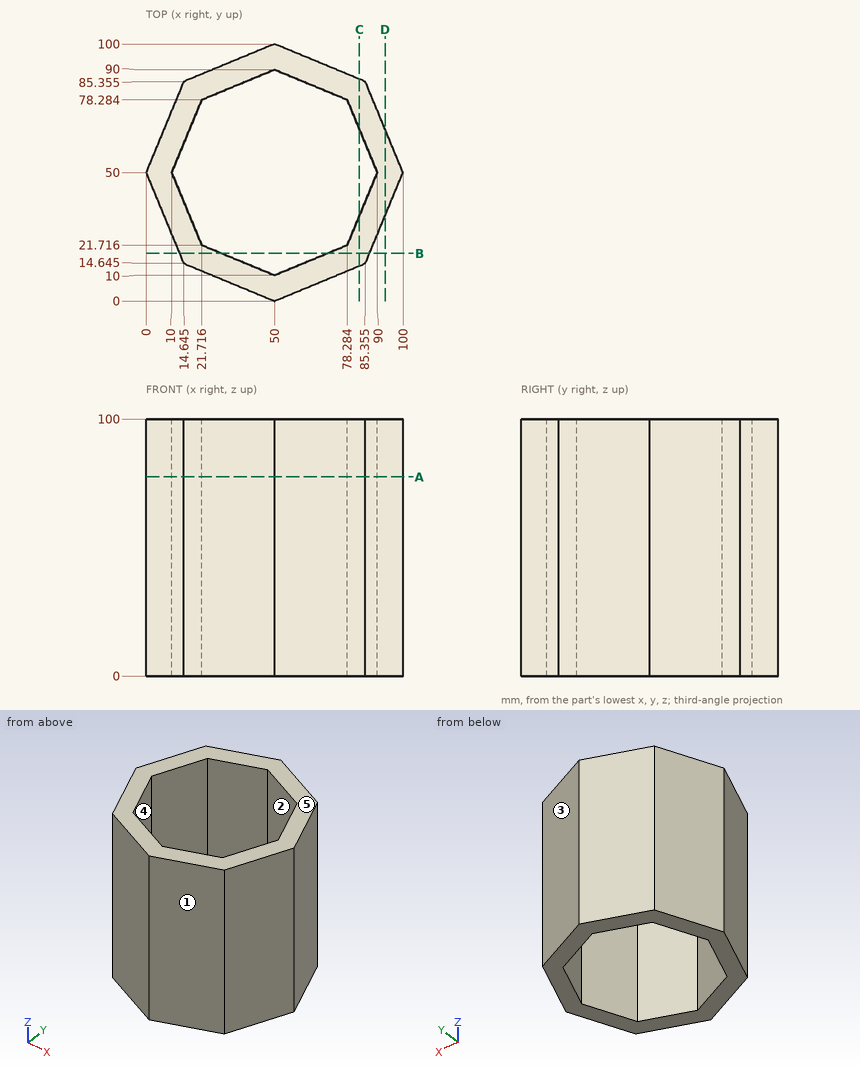
The drawing under review shows one solid part. Ordinate dimensions are in mm from its lowest x, y, z. A direction names the side the tool comes from. Round coordinates to 2 decimals unless told otherwise and drop trailing zeros. Loops run counter-clockwise (first coordinate to the right, second up) from the corner with the lowest first, then second, coordinate; pieces in that order, holes last. Notation, with made-up numbers: (15, 82.25) -> (20, 82.25) arc R23 ccw to (20, 101.25) -> close; hole circle Ø8 at (-11.75, 12). An arc over 180 degrees is marked (long way). Answer in a Markdown table with one row per item.
1) Consider section D-D, the plane x = 93. Write out the cut boundary in (y, z).
Taken from the geometry:
| item | result |
|---|---|
| outline | (33.1, 0) -> (66.9, 0) -> (66.9, 100) -> (33.1, 100) -> close |
2) Tool access review of the marked faces 1 and 2: name each direction out of +Z, -Z, +X, -X, +Y, -Y from which nothing blocks a thin tool from reaching the whole face with its end or side.
Taken from the geometry:
| item | result |
|---|---|
| face 1 | +Z, -Z, +X, -Y |
| face 2 | +Z, -Z |
3) Consider section C-C, the plane x = 83. Write out the cut boundary in (y, z).
Taken from the geometry:
| item | result |
|---|---|
| outline | (13.67, 0) -> (33.1, 0) -> (33.1, 100) -> (13.67, 100) -> close; (66.9, 0) -> (86.33, 0) -> (86.33, 100) -> (66.9, 100) -> close |
4) Consider section B-B, the plane y = 18.5. Write out the cut boundary in (x, z), plus the area to 3 significant figures.
Taken from the geometry:
| item | result |
|---|---|
| outline | (13.05, 0) -> (29.48, 0) -> (29.48, 100) -> (13.05, 100) -> close; (70.52, 0) -> (86.95, 0) -> (86.95, 100) -> (70.52, 100) -> close |
| area | 3,290 mm² |
5) Consider section A-A, the plane z = 77.5. Write out the cut boundary in (x, y) (1 decimal).
Taken from the geometry:
| item | result |
|---|---|
| outline | (0, 50) -> (14.6, 14.6) -> (50, 0) -> (85.4, 14.6) -> (100, 50) -> (85.4, 85.4) -> (50, 100) -> (14.6, 85.4) -> close; hole (10, 50) -> (21.7, 21.7) -> (50, 10) -> (78.3, 21.7) -> (90, 50) -> (78.3, 78.3) -> (50, 90) -> (21.7, 78.3) -> close |
6) Wall thickness on line 1 along Y through (x, z) = (37, 5.5) (1 decimal); line 2 along X through (y, z) = (48, 59); line 3 along Y through (x, z) = (13, 43.5) (1 decimal): over which ranges is each line inside the solid? List them lowest first.
Taken from the geometry:
| item | result |
|---|---|
| line 1 | y = 5.4 to 15.4, 84.6 to 94.6 |
| line 2 | x = 0.83 to 10.83, 89.17 to 99.17 |
| line 3 | y = 18.6 to 42.8, 57.2 to 81.4 |
7) Draft analysis for pull direction Y (two halves, no side actions). For the marked faces 3, 4 and 5, state which applies: pulls with the +Y half, pulls with the -Y half, needs draft (parallel to the pull), parting line crosses it, or undercut.
Taken from the geometry:
| item | result |
|---|---|
| face 3 | pulls with the +Y half |
| face 4 | undercut |
| face 5 | needs draft |
8) For pin 1 Ø8 at (x, z) = (18.5, 79.5) entering from +Y; pin 2 Ø1.5 at (x, z) = (41.5, 82.5) entering from -Y; pin 3 Ø1.5 at (y, z) = (86, 85.5) entering from +X, all flat-tipped, find the tip position at first contact; note any pin that passes through.
Taken from the geometry:
| item | result |
|---|---|
| pin 1 | stops at y = 88.61 |
| pin 2 | stops at y = 3.21 |
| pin 3 | stops at x = 85.4 |
